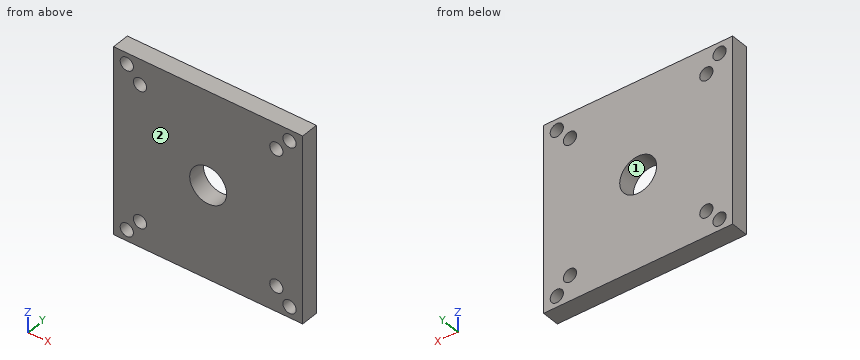
```python
from build123d import *

# Parameters (mm, degrees)
SKETCH_1_W          = 43
SKETCH_1_H          = 42.5
EXTRUDE_1_DEPTH     = 4
SKETCH_2_R          = 1.5
CUT_EXTRUDE_1_DEPTH = 10
SKETCH_3_R          = 1.5
CUT_EXTRUDE_2_DEPTH = 10
SKETCH_4_R          = 4.2
CUT_EXTRUDE_3_DEPTH = 4


with BuildPart() as part:
    # Эскиз1 → Бобышка-Вытянуть1 (new body)
    with BuildSketch(Plane(origin=(0, 0, 0), x_dir=(1, 0, 0), z_dir=(0, 1, 0))):
        with Locations((-15.064488683, 7.723245358)):
            Rectangle(SKETCH_1_W, SKETCH_1_H)
    extrude(amount=EXTRUDE_1_DEPTH)

    # Эскиз2 → Вырез-Вытянуть1 (cut)
    with BuildSketch(Plane.XZ):
        with Locations(Location((-33.564488683, 11.026754642, 0), (0, 0, 270))):
            Circle(SKETCH_2_R)
        with Locations(Location((3.435511317, 11.026754642, 0), (0, 0, 270))):
            Circle(SKETCH_2_R)
        with Locations(Location((-33.564488683, -26.473245358, 0), (0, 0, 270))):
            Circle(SKETCH_2_R)
        with Locations(Location((3.435511317, -26.473245358, 0), (0, 0, 270))):
            Circle(SKETCH_2_R)
    extrude(amount=-CUT_EXTRUDE_1_DEPTH, mode=Mode.SUBTRACT)

    # Эскиз3 → Вырез-Вытянуть2 (cut)
    with BuildSketch(Plane.XZ):
        with Locations(Location((-30.564488683, 7.776754642, 0), (0, 0, 270))):
            Circle(SKETCH_3_R)
        with Locations(Location((-30.564488683, -23.223245358, 0), (0, 0, 270))):
            Circle(SKETCH_3_R)
        with Locations(Location((0.435511317, 7.776754642, 0), (0, 0, 270))):
            Circle(SKETCH_3_R)
        with Locations(Location((0.435511317, -23.223245358, 0), (0, 0, 270))):
            Circle(SKETCH_3_R)
    extrude(amount=-CUT_EXTRUDE_2_DEPTH, mode=Mode.SUBTRACT)

    # Эскиз4 → Вырез-Вытянуть3 (cut)
    with BuildSketch(Plane(origin=(0, 4, 0), x_dir=(1, 0, 0), z_dir=(0, 1, 0))):
        with Locations(Location((-15.064488683, 7.723245358, 0), (0, 0, 270))):
            Circle(SKETCH_4_R)
    extrude(amount=-CUT_EXTRUDE_3_DEPTH, mode=Mode.SUBTRACT)


solid = part.part
```
Can you work these out from the model? Positions are in its coordinate system, mm. Face numbers are marked on the shaded views. Give positions to 0.01 mm unless a question says otherwise; leave off trailing zeros. Loops run counter-clockwise (first coordinate to the right, second up) from the corner with the lowest first, then second, coordinate; pieces in that order, holes last. Notation, with made-up numbers: M 24,84 L 61,84 A10 ccw 61,89 Z; hole C 24,27 d1. An arc over 180 degrees is marked long. One line per question, with ' | ' between items. Start each with the question number.
Q1. If we section it at D-D (x = 1): Please give me the cut outline in (y, z), plus the area to 3 significant figures.
Q2. If I drill on line 1 (X direction, y = 2.5, z = 11); line 2 (Z direction, x = -30.5, y = 1.5); line 3 (X direction, y = 3.05, z = 10), over which ranges is the centre line in solid material (lowest first)? Write a range as from..to.
Q3. If we section it at C-C (y = 2.4): State how many separate pieces and enclosed holes the cut face has, plus the area to 3 significant figures.
Q4. If we section it at B-B (z = -4.5): Please give me the cut outline in (x, y), plus the area to 3 significant figures.
Q5. If we section it at A-A (x = -14.5): Please give me the cut outline in (y, z).
Q6. If we mould it in two halves opening along X, with no side actions, what happens to the marked faces 1 and 2? For each: +X half, -X half, draft (parallel to the pull), parting line (faces both ways), or undercut.
Computed:
1) outline: M 0,-28.97 L 4,-28.97 L 4,-24.61 L 0,-24.61 Z; M 0,-21.83 L 4,-21.83 L 4,6.39 L 0,6.39 Z; M 0,9.17 L 4,9.17 L 4,13.53 L 0,13.53 Z | area: 148 mm²
2) line 1: x = -36.56..-35.06, -32.06..1.94, 4.94..6.44 | line 2: z = -28.97..-24.72, -21.72..6.28, 9.28..13.53 | line 3: x = -36.56..-34.66, -32.47..2.34, 4.53..6.44
3) separate pieces: 1 | enclosed holes: 9 | area: 1,720 mm²
4) outline: M -36.56,0 L -17.76,0 L -17.76,4 L -36.56,4 Z; M -12.37,0 L 6.44,0 L 6.44,4 L -12.37,4 Z | area: 150 mm²
5) outline: M 0,-28.97 L 4,-28.97 L 4,-11.89 L 0,-11.89 Z; M 0,-3.56 L 4,-3.56 L 4,13.53 L 0,13.53 Z
6) face 1: undercut | face 2: draft
